Source: CAD feature listing. Evaluate the final solid. Frame: model axes, mm. Face numbers are marked on the shaded views. A direction names the side the tool comes from. Round coordinates to 2 decimals unless told otherwise and drop trailing zeros. Write each loop counter-clockwise with the first axis right and the second up, starting at its lowest first coordinate (ties: lowest second). Pieces come first, ordered by that corner, then holes. Notation, with made-up numbers: M -2.75,-26.75 L 4.25,-26.75 A22 cw 4.25,9.25 Z; hole C 22,-33 d11. An arc over 180 degrees is marked long. Answer in a Markdown table with one row per item. Add a question column.
Item 1: Material intervals for probe 1 along Y at (x, z) = (50, 5); probe 2 along Y at (x, z) = (10, 3); probe 3 along Y at (x, z) = (30, 6.75), sorted ascending.
Item 2: Set-up query: the marked faces 1 and 2. Return all of +Z, -Z, +X, -X, +Y, -Y with unobstructed straight access to the full face (end or side cutting, diameter ignored); none if empty.
Item 3: Mould query, pull axis Y, two halves, no side actions, for the marked faces 3, 4, 5 and 6. Classes: released by +Y, released by -Y, zero draft, split by the parting line, or undercut.
Item 4: Contact query for flat-ended pins moving along their axis: pin 1 (1.5 mm diameter, centred on x = 12.5, y = 22, fed in from -Z); pin 2 (5 mm diameter, centred on y = 28.5, z = -7, fed in from +X). Output: stop coordinate, or through.
Item 5: Cut plane D-D on x = 30. Return loops of the section in (y, z), and give its area (3 significant figures).
Item 6: Cut plane B-B on x = 50. Return loops of the section in (y, z), and give its area (3 significant figures).
Item 7: Cut plane A-A on y = 50. Return loops of the section in (x, z), and give its area (3 significant figures).
Item 8: Cut plane C-C on z = -6. Return loops of the section in (x, y), and give its area (3 significant figures).
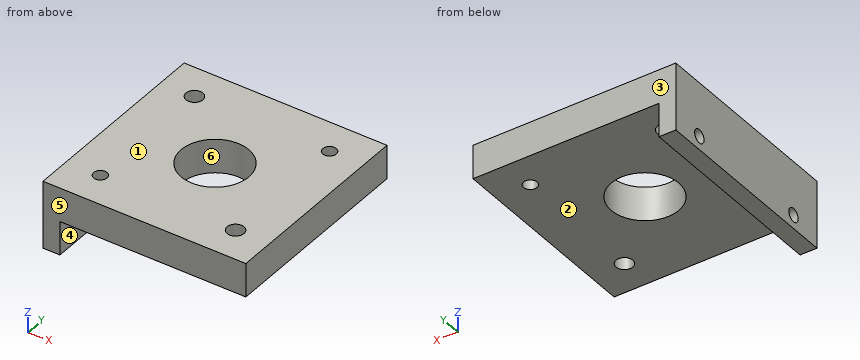
from build123d import *

# Parameters (mm, degrees)
SKETCH1_W           = 60
SKETCH1_H           = 60
BOSS_EXTRUDE1_DEPTH = 10
SKETCH4_W           = 5
SKETCH4_H           = 60
BOSS_EXTRUDE2_DEPTH = 10
SKETCH5_R           = 2
CUT_EXTRUDE3_DEPTH  = 86.440037453
SKETCH2_R           = 10
CUT_EXTRUDE5_DEPTH  = 86.440037453
CAVITY1_OUTLINE_R   = 2.5
CAVITY1_DEPTH       = 10
SKETCH7_R           = 2
CUT_EXTRUDE6_DEPTH  = 88.177978871


# Read off the part's stored shape, not the designer's step: Cavity1
with BuildPart() as part:
    # Sketch1 → Boss-Extrude1 (new body)
    with BuildSketch(Plane.XY):
        with Locations((30, 30)):
            Rectangle(SKETCH1_W, SKETCH1_H)
    extrude(amount=BOSS_EXTRUDE1_DEPTH)

    # Sketch4 → Boss-Extrude2 (add)
    with BuildSketch(Plane(origin=(0, 0, 0), x_dir=(-1, 0, 0), z_dir=(0, 0, -1))):
        with Locations((-2.5, 30)):
            Rectangle(SKETCH4_W, SKETCH4_H)
    extrude(amount=BOSS_EXTRUDE2_DEPTH)

    # Sketch5 → Cut-Extrude3 (cut, through all)
    with BuildSketch(Plane.ZY):
        with Locations((-6, 50)):
            Circle(SKETCH5_R)
        with Locations((-6, 10)):
            Circle(SKETCH5_R)
    extrude(amount=-CUT_EXTRUDE3_DEPTH, mode=Mode.SUBTRACT)

    # Sketch2 → Cut-Extrude5 (cut, through all)
    with BuildSketch(Plane(origin=(0, 0, 0), x_dir=(-1, 0, 0), z_dir=(0, 0, -1))):
        with Locations((-30, 30)):
            Circle(SKETCH2_R)
    extrude(amount=-CUT_EXTRUDE5_DEPTH, mode=Mode.SUBTRACT)

    # Cavity1 outline → Cavity1 (cut)
    with BuildSketch(Plane.XY):
        with Locations((10, 50)):
            Circle(CAVITY1_OUTLINE_R)
        with Locations((50, 10)):
            Circle(CAVITY1_OUTLINE_R)
    extrude(amount=CAVITY1_DEPTH, mode=Mode.SUBTRACT)

    # Sketch7 → Cut-Extrude6 (cut, through all)
    with BuildSketch(Plane.XY.offset(10)):
        with Locations((50, 50)):
            Circle(SKETCH7_R)
        with Locations((10, 10)):
            Circle(SKETCH7_R)
    extrude(amount=-CUT_EXTRUDE6_DEPTH, mode=Mode.SUBTRACT)


solid = part.part
Results below:
| question | item | result |
|---|---|---|
| 1 | probe 1 | 0 to 7.5, 12.5 to 48, 52 to 60 |
| 1 | probe 2 | 0 to 8, 12 to 47.5, 52.5 to 60 |
| 1 | probe 3 | 0 to 20, 40 to 60 |
| 2 | face 1 | +Z, +X, -X, +Y, -Y |
| 2 | face 2 | -Z, +X, +Y, -Y |
| 3 | face 3 | released by +Y |
| 3 | face 4 | zero draft |
| 3 | face 5 | released by -Y |
| 3 | face 6 | undercut |
| 4 | pin 1 | z = 0 |
| 4 | pin 2 | x = 5 |
| 5 | outline | M 0,0 L 20,0 L 20,10 L 0,10 Z; M 40,0 L 60,0 L 60,10 L 40,10 Z |
| 5 | area | 400 mm2 |
| 6 | outline | M 0,0 L 7.5,0 L 7.5,10 L 0,10 Z; M 12.5,0 L 48,0 L 48,10 L 12.5,10 Z; M 52,0 L 60,0 L 60,10 L 52,10 Z |
| 6 | area | 510 mm2 |
| 7 | outline | M 0,-10 L 5,-10 L 5,-8 L 0,-8 Z; M 0,-4 L 5,-4 L 5,0 L 7.5,0 L 7.5,10 L 0,10 Z; M 12.5,0 L 48,0 L 48,10 L 12.5,10 Z; M 52,0 L 60,0 L 60,10 L 52,10 Z |
| 7 | area | 540 mm2 |
| 8 | outline | M 0,0 L 5,0 L 5,8 L 0,8 Z; M 0,12 L 5,12 L 5,48 L 0,48 Z; M 0,52 L 5,52 L 5,60 L 0,60 Z |
| 8 | area | 260 mm2 |
